Can you work these out from the model? Positions are in its coordinate system, mm. Face numbers are marked on the shaded views. Give positions to 0.01 mm unless a question says otherwise; leave off trailing zeros. Loops run counter-clockwise (first coordinate to the right, second up) from the corner with the lowest first, then second, coordinate; pieces in that order, holes last. Notation, with made-up numbers: M 44.5,-30.75 L 66.5,-30.75 A12 cw 66.5,-21.75 Z; hole C -3.5,-25 d3. An arc over 180 degrees is marked long. Answer as a JSON object with one key per item and string values.
```python
from build123d import *

# Parameters (mm, degrees)
BOSS_EXTRUDE1_DEPTH = 50.8
SKETCH2_R           = 9.525
CUT_EXTRUDE1_DEPTH  = 50.8
SKETCH3_R           = 1.4224
CUT_EXTRUDE2_DEPTH  = 67.675


with BuildPart() as part:
    # Sketch1 → Boss-Extrude1 (new body)
    with BuildSketch(Plane.XY):
        Polygon((25.4, 0), (0, 0), (0, 38.1), (3.175, 38.1), (3.175, 3.175), (25.4, 3.175), align=None)
    extrude(amount=BOSS_EXTRUDE1_DEPTH)

    # Sketch2 → Cut-Extrude1 (cut)
    with BuildSketch(Plane(origin=(3.175, 0, 0), x_dir=(0, 0, -1), z_dir=(1, 0, 0))):
        with Locations(Location((-25.4, 20.6375, 0), (0, 0, 90))):
            Circle(SKETCH2_R)
    extrude(amount=-CUT_EXTRUDE1_DEPTH, mode=Mode.SUBTRACT)

    # Sketch3 → Cut-Extrude2 (cut, through all)
    with BuildSketch(Plane(origin=(0, 3.175, 0), x_dir=(1, 0, 0), z_dir=(0, 1, 0))):
        with Locations(Location((14.2875, -11.1125, 0), (0, 0, 270))):
            Circle(SKETCH3_R)
        with Locations(Location((14.2875, -39.6875, 0), (0, 0, 270))):
            Circle(SKETCH3_R)
    extrude(amount=-CUT_EXTRUDE2_DEPTH, mode=Mode.SUBTRACT)


solid = part.part
```
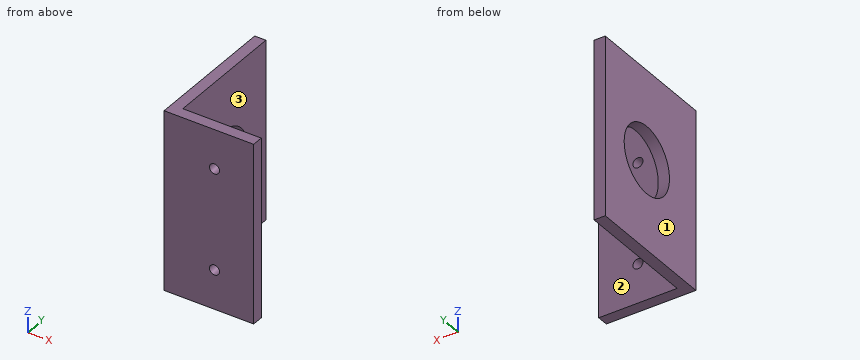
1) Suppose I cut it at D-D, the plane z = 36. Write out the boundary of the cut face in (x, y) (3 decimals), and give its area (3 significant figures).
Answer list:
{"outline": "M 0,0 L 25.4,0 L 25.4,3.175 L 3.175,3.175 L 3.175,38.1 L 0,38.1 Z", "area": "192 mm^2"}
2) If we mould it in two halves opening along X, with no side actions, what happens to the marked faces 1, 2 and 3? For each: +X half, -X half, draft (parallel to the pull), parting line (faces both ways), or undercut.
Answer list:
{"face 1": "-X half", "face 2": "draft", "face 3": "+X half"}
3) Please list where these lines run through material, in increasing order: line 1 along X through (y, z) = (3.5, 23) (3 decimals); line 2 along Y through (x, z) = (2.25, 20.5). Write a range as from..to.
Answer list:
{"line 1": "0..3.175", "line 2": "0..12.47, 28.81..38.1"}
4) Will these pins go through, and if not, where does the flat tip stop? pin 1 Ø10 at (y, z) = (24.5, 15) entering from +X (3 decimals); pin 2 Ø6.5 at (x, z) = (14.5, 24) entering from +Y (3 decimals).
Answer list:
{"pin 1": "x = 3.175", "pin 2": "y = 3.175"}
5) Suppose I cut it at A-A, the plane z = 25.4. Write out the boundary of the cut face in (x, y) (1 decimal), and give its area (3 significant figures).
Answer list:
{"outline": "M 0,0 L 25.4,0 L 25.4,3.2 L 3.2,3.2 L 3.2,11.1 L 0,11.1 Z; M 0,30.2 L 3.2,30.2 L 3.2,38.1 L 0,38.1 Z", "area": "131 mm^2"}
6) Suppose I cut it at B-B, the plane y = 21. Write out the boundary of the cut face in (x, z) (3 decimals).
Answer list:
{"outline": "M 0,0 L 3.175,0 L 3.175,15.882 L 0,15.882 Z; M 0,34.918 L 3.175,34.918 L 3.175,50.8 L 0,50.8 Z"}
7) Suppose I cut it at C-C, the plane x = 13.5. Write out the boundary of the cut face in (y, z) (3 decimals).
Answer list:
{"outline": "M 0,0 L 3.175,0 L 3.175,9.928 L 0,9.928 Z; M 0,12.297 L 3.175,12.297 L 3.175,38.503 L 0,38.503 Z; M 0,40.872 L 3.175,40.872 L 3.175,50.8 L 0,50.8 Z"}
